```python
from build123d import *

# Parameters (mm, degrees)
SKETCH1_W           = 30
SKETCH1_H           = 16
BOSS_EXTRUDE1_DEPTH = 20
CUT_EXTRUDE1_DEPTH  = 20
SKETCH3_W           = 6
SKETCH3_H           = 10
BOSS_EXTRUDE2_DEPTH = 5
SKETCH9_R           = 1.6
CUT_EXTRUDE3_DEPTH  = 4.5
SKETCH11_W          = 10
SKETCH11_H          = 8
BOSS_EXTRUDE4_DEPTH = 40
CHAMFER2_SIZE2      = 10
CHAMFER2_SIZE       = 2
FILLET1_R           = 1
CUT_EXTRUDE4_DEPTH  = 8
SKETCH13_W          = 2
SKETCH13_H          = 8
BOSS_EXTRUDE5_DEPTH = 10
LPATTERN1_COUNT     = 8
LPATTERN1_PITCH     = 4.25
FILLET2_R           = 0.5
FILLET3_R           = 1
SKETCH14_W          = 2
SKETCH14_H          = 8
CUT_EXTRUDE5_DEPTH  = 17
CHAMFER9_SIZE       = 5
SKETCH15_W          = 19.120114905
SKETCH15_H          = 8.62957368
CUT_EXTRUDE6_DEPTH  = 1


# Some blends are built 0.0001 mm under size
with BuildPart() as part:
    # Sketch1 → Boss-Extrude1 (new body)
    with BuildSketch(Plane.XY):
        with Locations((15, -8)):
            Rectangle(SKETCH1_W, SKETCH1_H)
    extrude(amount=BOSS_EXTRUDE1_DEPTH)

    # Sketch2 → Cut-Extrude1 (cut)
    with BuildSketch(Plane.XY.offset(20)):
        Polygon((22, -4.5), (22, -7.5), (30, -7.5), (30, -16), (5, -16), (5, -4.5), align=None)
    extrude(amount=-CUT_EXTRUDE1_DEPTH, mode=Mode.SUBTRACT)

    # Sketch3 → Boss-Extrude2 (add)
    with BuildSketch(Plane.XZ.offset(16)):
        with Locations((3, 10)):
            Rectangle(SKETCH3_W, SKETCH3_H)
    extrude(amount=BOSS_EXTRUDE2_DEPTH)

    # Sketch9 → Cut-Extrude3 (cut)
    with BuildSketch(Plane.XZ.offset(4.5)):
        with Locations(Location((18, 15, 0), (0, 0, 270))):
            Circle(SKETCH9_R)
        with Locations(Location((18, 5, 0), (0, 0, 270))):
            Circle(SKETCH9_R)
    extrude(amount=-CUT_EXTRUDE3_DEPTH, mode=Mode.SUBTRACT)

    # Sketch11 → Boss-Extrude4 (add)
    with BuildSketch(Plane.XY.offset(15)):
        with Locations((3, -17)):
            Rectangle(SKETCH11_W, SKETCH11_H)
    extrude(amount=BOSS_EXTRUDE4_DEPTH)

    # Chamfer2
    chamfer2_edges = [part.edges().sort_by_distance(p)[0] for p in [
        (0, -17, 15),
    ]]
    chamfer2_side = [part.faces().sort_by_distance(p)[0] for p in [
        (-0.04, -17, 15),
    ]]
    chamfer(chamfer2_edges, length=CHAMFER2_SIZE - 0.0001, length2=CHAMFER2_SIZE2 - 0.0001, reference=chamfer2_side[0])  # a hair under: the kernel refuses the full size

    # Fillet1
    fillet1_edges = [part.edges().sort_by_distance(p)[0] for p in [
        (2.5, -13, 20),
    ]]
    fillet(fillet1_edges, radius=FILLET1_R)

    # Sketch12 → Cut-Extrude4 (cut)
    with BuildSketch(Plane.XZ.offset(21)):
        Polygon((6.5, 55), (4.25, 54.5), (2, 53.75), (2, 52.75), (4.25, 52), (6.5, 51.5), (6.5, 50.75), (8, 50.75), (8, 55), align=None)
    cut_extrude4 = extrude(amount=-CUT_EXTRUDE4_DEPTH, mode=Mode.SUBTRACT)

    # Sketch13 → Boss-Extrude5 (add)
    with BuildSketch(Plane(origin=(0, 0, 15), x_dir=(-1, 0, 0), z_dir=(0, 0, -1))):
        with Locations((-7, -17)):
            Rectangle(SKETCH13_W, SKETCH13_H)
    extrude(amount=BOSS_EXTRUDE5_DEPTH)

    # LPattern1: Cut-Extrude4 ×8
    with Locations(*[(0, 0, -i * LPATTERN1_PITCH) for i in range(1, LPATTERN1_COUNT)]):
        add(cut_extrude4, mode=Mode.SUBTRACT)

    # Fillet2
    # the kernel refuses this fillet: 0.5 mm, written as the material it adds along each edge
    with BuildSketch(Plane(origin=(2, -21, 52.75), x_dir=(0.9486832980505142, 0, -0.31622776601683683), z_dir=(0, 1, 0)), Plane(origin=(2, -21, 53.75), x_dir=(0, 0, -1), z_dir=(0, 1, 0)), Plane(origin=(2, -21, 48.5), x_dir=(0.9486832980505137, 0, -0.31622776601683833), z_dir=(0, 1, 0)), Plane(origin=(2, -21, 49.5), x_dir=(0, 0, -1), z_dir=(0, 1, 0)), Plane(origin=(2, -21, 44.25), x_dir=(0.9486832980505137, 0, -0.31622776601683833), z_dir=(0, 1, 0)), Plane(origin=(2, -21, 45.25), x_dir=(0, 0, -1), z_dir=(0, 1, 0)), Plane(origin=(2, -21, 35.75), x_dir=(0.9486832980505137, 0, -0.31622776601683833), z_dir=(0, 1, 0)), Plane(origin=(2, -21, 36.75), x_dir=(0, 0, -1), z_dir=(0, 1, 0)), Plane(origin=(2, -21, 40), x_dir=(0.9486832980505137, 0, -0.31622776601683833), z_dir=(0, 1, 0)), Plane(origin=(2, -21, 41), x_dir=(0, 0, -1), z_dir=(0, 1, 0)), Plane(origin=(2, -21, 23), x_dir=(0.9486832980505137, 0, -0.31622776601683833), z_dir=(0, 1, 0)), Plane(origin=(2, -21, 24), x_dir=(0, 0, -1), z_dir=(0, 1, 0)), Plane(origin=(2, -21, 27.25), x_dir=(0.9486832980505137, 0, -0.31622776601683833), z_dir=(0, 1, 0)), Plane(origin=(2, -21, 28.25), x_dir=(0, 0, -1), z_dir=(0, 1, 0)), Plane(origin=(2, -21, 32.5), x_dir=(0, 0, -1), z_dir=(0, 1, 0)), Plane(origin=(2, -21, 31.5), x_dir=(0.9486832980505137, 0, -0.31622776601683833), z_dir=(0, 1, 0))) as fillet2_piece_1:
        with BuildLine():
            CenterArc((FILLET2_R * 0.720759220056, -FILLET2_R), FILLET2_R, 90, 71.565051177)
            Line((-FILLET2_R * 0.227924077994, -FILLET2_R * 0.683772233983), (0, 0))
            Line((0, 0), (FILLET2_R * 0.720759220056, 0))
        make_face()
    extrude(amount=8)
    # the kernel refuses this fillet: 0.5 mm, written as the material it takes off along each edge
    with BuildSketch(Plane(origin=(6.5, -22.002714508, 33.75), x_dir=(-0.9761870601839537, 0, -0.21693045781865147), z_dir=(0, 1, 0)), Plane(origin=(6.5, -22.002714508, 34.5), x_dir=(0, 0, -1), z_dir=(0, 1, 0)), Plane(origin=(6.5, -22.002714508, 38), x_dir=(-0.9761870601839536, 0, -0.21693045781865192), z_dir=(0, 1, 0)), Plane(origin=(6.5, -22.002714508, 38.75), x_dir=(0, 0, -1), z_dir=(0, 1, 0)), Plane(origin=(6.5, -22.002714508, 42.25), x_dir=(-0.9761870601839541, 0, -0.21693045781865056), z_dir=(0, 1, 0)), Plane(origin=(6.5, -22.002714508, 43), x_dir=(0, 0, -1), z_dir=(0, 1, 0)), Plane(origin=(6.5, -22.002714508, 46.5), x_dir=(-0.9761870601839537, 0, -0.21693045781865147), z_dir=(0, 1, 0)), Plane(origin=(6.5, -22.002714508, 47.25), x_dir=(0, 0, -1), z_dir=(0, 1, 0)), Plane(origin=(6.5, -22.002714508, 50.75), x_dir=(-0.9761870601839541, 0, -0.21693045781865006), z_dir=(0, 1, 0)), Plane(origin=(6.5, -22.002714508, 51.5), x_dir=(0, 0, -1), z_dir=(0, 1, 0)), Plane(origin=(6.5, -22.002714508, 25.25), x_dir=(-0.9761870601839524, 0, -0.21693045781865805), z_dir=(0, 1, 0)), Plane(origin=(6.5, -22.002714508, 26), x_dir=(0, 0, -1), z_dir=(0, 1, 0)), Plane(origin=(6.5, -22.002714508, 29.5), x_dir=(-0.9761870601839522, 0, -0.216930457818659), z_dir=(0, 1, 0)), Plane(origin=(6.5, -22.002714508, 30.25), x_dir=(0, 0, -1), z_dir=(0, 1, 0))) as fillet2_2_piece_1:
        with BuildLine():
            CenterArc((FILLET2_R * 0.802171606366, FILLET2_R), FILLET2_R, 192.528807709, 77.471192291)
            Line((-FILLET2_R * 0.174015453818, FILLET2_R * 0.783069542181), (0, 0))
            Line((0, 0), (FILLET2_R * 0.802171606366, 0))
        make_face()
    extrude(amount=10.005429016, mode=Mode.SUBTRACT)

    # Fillet3
    # the kernel refuses this fillet: 1 mm, written as the material it takes off along each edge
    with BuildSketch(Plane(origin=(6.5, -28.790063509, 55), x_dir=(-1, 0, 0), z_dir=(0, 1, 0))) as fillet3_piece_1:
        with BuildLine():
            CenterArc((3.116025404, -1), FILLET3_R, 90, 60)
            Line((2.25, -0.5), (0, 0))
            Line((0, 0), (3.116025404, 0))
        make_face()
    extrude(amount=23.580127019, mode=Mode.SUBTRACT)

    # Sketch14 → Cut-Extrude5 (cut)
    with BuildSketch(Plane(origin=(0, 0, 5), x_dir=(-1, 0, 0), z_dir=(0, 0, -1))):
        with Locations((-7, -17)):
            Rectangle(SKETCH14_W, SKETCH14_H)
    extrude(amount=-CUT_EXTRUDE5_DEPTH, mode=Mode.SUBTRACT)

    # Chamfer9
    # the kernel refuses this chamfer: 5 mm, written as the material it takes off along each edge
    with BuildSketch(Plane(origin=(5, -16, 17.85841494), x_dir=(0, 1, 0), z_dir=(0, 0, -1))) as chamfer9_piece_1_section:
        Polygon((CHAMFER9_SIZE, 0), (0, -CHAMFER9_SIZE), (0, 0), align=None)
    chamfer9_piece_1 = extrude(amount=30.71682988, mode=Mode.PRIVATE)
    chamfer9_piece_1 = split(chamfer9_piece_1, bisect_by=Plane(origin=(5, -22.42920747, 11.42920747), z_dir=(0, -0.7071067811865476, -0.7071067811865476)), keep=Keep.TOP, mode=Mode.PRIVATE)
    add(chamfer9_piece_1, mode=Mode.SUBTRACT)
    with BuildSketch(Plane(origin=(0, -16, -12.85841494), x_dir=(0, 1, 0), z_dir=(0, 0, 1))) as chamfer9_piece_2_section:
        Polygon((CHAMFER9_SIZE, 0), (0, -CHAMFER9_SIZE), (0, 0), align=None)
    chamfer9_piece_2 = extrude(amount=30.71682988, mode=Mode.PRIVATE)
    chamfer9_piece_2 = split(chamfer9_piece_2, bisect_by=Plane(origin=(0, -7.07079253, -3.92920747), z_dir=(0, -0.7071067811865476, -0.7071067811865476)), keep=Keep.TOP, mode=Mode.PRIVATE)
    add(chamfer9_piece_2, mode=Mode.SUBTRACT)
    with BuildSketch(Plane(origin=(0, -3.14158506, 5), x_dir=(1, 0, 0), z_dir=(0, -1, 0))) as chamfer9_piece_3_section:
        Polygon((CHAMFER9_SIZE, 0), (0, CHAMFER9_SIZE), (0, 0), align=None)
    chamfer9_piece_3 = extrude(amount=30.71682988, mode=Mode.PRIVATE)
    chamfer9_piece_3 = split(chamfer9_piece_3, bisect_by=Plane(origin=(0, -9.57079253, -1.42920747), z_dir=(0, -0.707106781186547, -0.7071067811865481)), keep=Keep.TOP, mode=Mode.PRIVATE)
    add(chamfer9_piece_3, mode=Mode.SUBTRACT)
    with BuildSketch(Plane(origin=(18.85841494, -21, 5), x_dir=(0, 0, 1), z_dir=(-1, 0, 0))) as chamfer9_piece_4:
        Polygon((CHAMFER9_SIZE, 0), (0, CHAMFER9_SIZE), (0, 0), align=None)
    extrude(amount=31.71682988, mode=Mode.SUBTRACT)
    with BuildSketch(Plane(origin=(6, -33.85841494, 5), x_dir=(0, 0, 1), z_dir=(0, 1, 0))) as chamfer9_piece_5_section:
        Polygon((CHAMFER9_SIZE, 0), (0, -CHAMFER9_SIZE), (0, 0), align=None)
    chamfer9_piece_5 = extrude(amount=30.71682988, mode=Mode.PRIVATE)
    chamfer9_piece_5 = split(chamfer9_piece_5, bisect_by=Plane(origin=(6, -24.92920747, 13.92920747), z_dir=(0, -0.707106781186547, -0.7071067811865481)), keep=Keep.TOP, mode=Mode.PRIVATE)
    add(chamfer9_piece_5, mode=Mode.SUBTRACT)
    with BuildSketch(Plane(origin=(17.85841494, -16, 0), x_dir=(0, 0, 1), z_dir=(-1, 0, 0))) as chamfer9_piece_6:
        Polygon((CHAMFER9_SIZE, 0), (0, CHAMFER9_SIZE), (0, 0), align=None)
    extrude(amount=30.71682988, mode=Mode.SUBTRACT)

    # Sketch15 → Cut-Extrude6 (cut)
    with BuildSketch(Plane(origin=(6, 0, 0), x_dir=(0, 0, -1), z_dir=(1, 0, 0))):
        with Locations((-12.83373262, -16.68521316)):
            Rectangle(SKETCH15_W, SKETCH15_H)
    extrude(amount=-CUT_EXTRUDE6_DEPTH, mode=Mode.SUBTRACT)


solid = part.part
```
Input: part model. Units: mm. Frame: model coordinates. A direction names the side the tool comes from. Round coordinates to 2 decimals unless told otherwise and drop trailing zeros. Write each loop counter-clockwise with the first axis right and the second up, starting at its lowest first coordinate (ties: lowest second). Pieces come first, ordered by that corner, then holes. Notation, with made-up numbers: (51.25, -11) -> (100.25, -11) arc R21 ccw to (100.25, 25) -> close; hole circle Ø9 at (65.25, 43.25). An arc over 180 degrees is marked (long way). Answer as CSV lines item,"result".
1. Ray query, L1, parallel to X at y = -7, z = 7.5; L2, parallel to X at y = -1.95, z = 5; L3, parallel to Z at x = 1, y = -8. Return the intervals inside material, ascending. Write a range as [from, to].
Geometry says:
L1,"x = [0, 5], [22, 30]"
L2,"x = [0, 16.4], [19.6, 30]"
L3,"z = [0, 20]"
2. Section A-A (x = 18). Return the cut outline in (y, z), plus the area to 3 significant figures.
Geometry says:
outline,"(-4.5, 0) -> (0, 0) -> (0, 3.4) -> (-4.5, 3.4) -> close; (-4.5, 6.6) -> (0, 6.6) -> (0, 13.4) -> (-4.5, 13.4) -> close; (-4.5, 16.6) -> (0, 16.6) -> (0, 20) -> (-4.5, 20) -> close"
area,"61.2 mm^2"
3. Section D-D (x = 9). Return the cut outline in (y, z), plus the area to 3 significant figures.
Geometry says:
outline,"(-4.5, 0) -> (0, 0) -> (0, 20) -> (-4.5, 20) -> close"
area,"90.0 mm^2"
4. Section B-B (y = -2.5). Return the cut outline in (x, z), plus the area to 3 significant figures.
Geometry says:
outline,"(0, 0) -> (30, 0) -> (30, 20) -> (0, 20) -> close; hole circle Ø3.2 at (18, 5); hole circle Ø3.2 at (18, 15)"
area,"584 mm^2"
5. Reachability of faces 4 (the cylindrical face through (19.586, -2.282, 5.208)), 5 (the flat face through (3.283, -17.056, 39.572)) from +Z, -Z, +X, -X, +Y, -Y: full face, straight path, thin tool, end or side. Return the list, or none.
Geometry says:
face 4,"+Y, -Y"
face 5,"+X, +Y, -Y"
6. Section C-C (z = 9). Return the cut outline in (x, y), plus the area to 3 significant figures.
Geometry says:
outline,"(-0.8, -20) -> (5, -20) -> (5, -4.5) -> (22, -4.5) -> (22, -7.5) -> (30, -7.5) -> (30, 0) -> (0, 0) -> (0, -13) -> (-0.8, -13) -> close"
area,"242 mm^2"
7. Mould query, pull axis X, two halves, no side actions, for faces 1 (the flat face through (5.166, -17.056, 39.046)), 2 (the flat face through (5, -13, 11)), 3 (the flat face through (2, -16, 5)). Classes: +X half, -X half, draft (parallel to the pull), parting line (faces both ways), or undercut.
Geometry says:
face 1,"+X half"
face 2,"undercut"
face 3,"draft"
8. Contact query for flat-ended pins moving along their axis: P1, Ø5, axis at x = 6, z = 47.5, coming from the +Y side; P2, Ø3, axis at x = 18.5, y = -2.5, coming from the +Z side; P3, Ø5, axis at y = -7.5, z = 9, coming from the -X side; P4, Ø1.9, axis at x = 18, z = 15, coming from the -Y side. Output: stop coordinate, or through.
Geometry says:
P1,"stops at y = -13"
P2,"stops at z = 20"
P3,"stops at x = 0"
P4,"passes through"
